Can you work these out from the model? Positions are in its coordinate system, mm. Face numbers are marked on the shaded views. Coordinates: 2 decimals unless noted, no trailing zeros. Order: outer loops, then holes, each group sorted by start corner. A loop starts at its lowest first (then second) coordinate and runs counter-clockwise, first axis right, second up. Notation, with made-up numbers: (21.5, 83) - (35.5, 83) arc R15 ccw to (35.5, 100) - close; hole circle Ø8 at (-12.5, 72.25). An arc over 180 degrees is marked (long way). Return JSON: item names as keys, results as strings. Group by question number.
1) Imagine slicing it at A-A (x = 0). Write out the boundary of the cut face in (y, z) (1 decimal).
2) If I drill on line 1 along Y through (x, z) = (-1, 17.25); line 2 along X through (y, z) = (-7.5, 4); line 3 along Y through (x, z) = (-24.5, 12.25), over which ranges is the centre line in solid material (lowest first)?
3) If we mould it in two halves opening along Y, with no side actions, what happens to the marked faces 1, 2, 3 and 4? For each: pulls with the +Y half, pulls with the -Y half, needs draft (parallel to the pull), parting line crosses it, or undercut.
4) Imagine slicing it at D-D (y = -36). Write out the boundary of the cut face in (x, z) (3 decimals).
5) For pin 1 Ø6 at (x, z) = (29.5, 9.5) entering from +Y; pin 2 Ø8 at (x, y) = (-27.5, 3.5) entering from +Z, each with a flat end and sliding along its axis, tell me the tip position at first contact or that it passes through.
6) Imagine slicing it at C-C (z = 6.5). Give the number of separate pieces and of enclosed holes in the cut face, and give its area (3 significant figures).
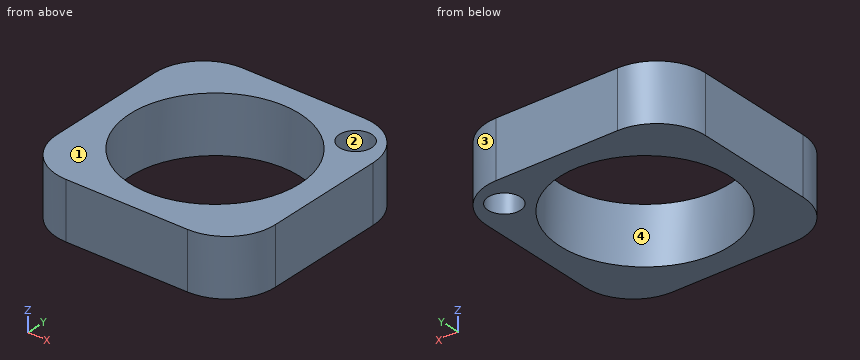
```python
from build123d import *

# Parameters (mm, degrees)
F0_R     = 33.3375
F0_R_2   = 6.35
F1_DEPTH = 22.225


with BuildPart() as f1:
    # F0 (on Top) → F1 (new body)
    with BuildSketch(Plane.XY):
        with BuildLine():
            ThreePointArc((-42.8625, -23.8125), (-37.282884, -37.282884), (-23.8125, -42.8625))
            Line((-23.8125, -42.8625), (23.8125, -42.8625))
            ThreePointArc((23.8125, -42.8625), (37.282884, -37.282884), (42.8625, -23.8125))
            Line((42.8625, -23.8125), (42.8625, 23.8125))
            ThreePointArc((42.8625, 23.8125), (37.282884, 37.282884), (23.8125, 42.8625))
            Line((23.8125, 42.8625), (-23.8125, 42.8625))
            ThreePointArc((-23.8125, 42.8625), (-37.282884, 37.282884), (-42.8625, 23.8125))
            Line((-42.8625, 23.8125), (-42.8625, -23.8125))
        make_face()
        Circle(F0_R, mode=Mode.SUBTRACT)
        with Locations((30.547692, 30.547692)):
            Circle(F0_R_2, mode=Mode.SUBTRACT)
    extrude(amount=F1_DEPTH)


solid = f1.part
```
Calculated:
{
 "1": {"outline": "(-42.9, 0) - (-33.3, 0) - (-33.3, 22.2) - (-42.9, 22.2) - close; (33.3, 0) - (42.9, 0) - (42.9, 22.2) - (33.3, 22.2) - close"},
 "2": {"line 1": "-42.86 to -33.32, 33.32 to 42.86", "line 2": "-42.86 to -32.48, 32.48 to 42.86", "line 3": "-42.85 to -22.61, 22.61 to 42.85"},
 "3": {"face 1": "needs draft", "face 2": "undercut", "face 3": "pulls with the +Y half", "face 4": "undercut"},
 "4": {"outline": "(-38.454, 0) - (38.454, 0) - (38.454, 22.225) - (-38.454, 22.225) - close"},
 "5": {"pin 1": "y = 42.67", "pin 2": "through"},
 "6": {"separate pieces": "1", "enclosed holes": "2", "area": "3,420 mm2"}
}
